Geometry: see drawing. Coordinates: mm, zero at the bounding-box minimum. A direction names the side the tool comes from. Coordinates: 2 decimals unless noted, no trailing zeros. Write each loop counter-clockwise with the first axis right and the second up, starting at its lowest first coordinate (ties: lowest second). Pieces come first, ordered by that corner, then holes.
1) Section query B-B (x = 16). Output: boundary loops of the cut face in (y, z) (1 decimal), then the cut area to 3 significant figures.
2) Section query A-A (z = 13). Output: boundary loops of the cut face in (x, y) (1 decimal).
3) Pin query (flat end, axial travel): pin 1 Ø10 at (y, z) = (96, 25) entering from +X; pin 2 Ø12 at (x, y) = (5, 98) entering from +Z (1 decimal); pin 3 Ø12 at (y, z) = (90.5, 12) entering from -X. Return the tip coordinate at first contact, or that it passes through.
4) Section query C-C (y = 111.5). Output: boundary loops of the cut face in (x, z), then the cut area to 3 significant figures.
5) Line query: L1, parallel to Y at x = 30, z = 30.5 (1 decimal); L2, parallel to X at y = 35.5, z = 25.5 (1 decimal); L3, parallel to X at y = 111, z = 22 (1 decimal). Output: solid intervals per line, ascending.
6) Set-up query: the marked faces 1 and 2. Return all of +Z, -Z, +X, -X, +Y, -Y with unobstructed straight access to the full face (end or side cutting, diameter ignored); none if empty.
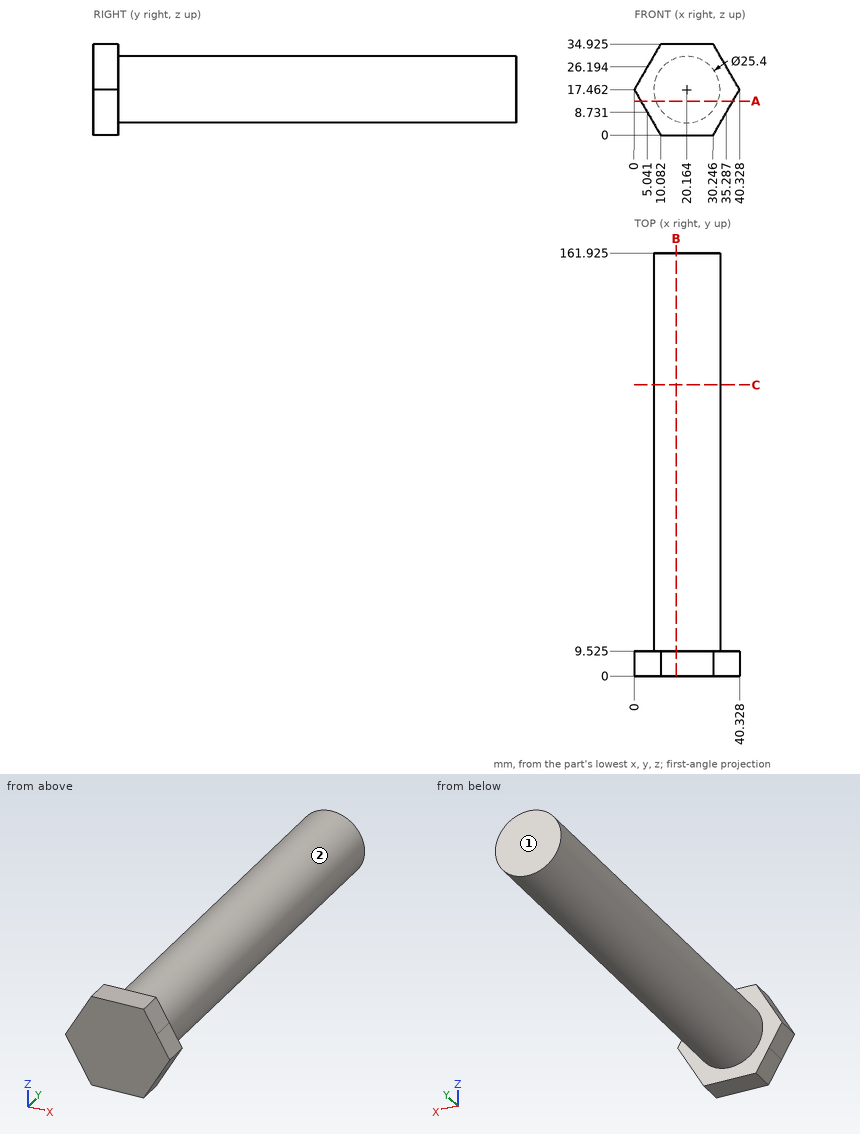
Answer:
1. outline: (0, 0) - (9.5, 0) - (9.5, 5.5) - (161.9, 5.5) - (161.9, 29.5) - (9.5, 29.5) - (9.5, 34.9) - (0, 34.9) - close
1. area: 3,990 mm2
2. outline: (2.6, 0) - (37.8, 0) - (37.8, 9.5) - (32.1, 9.5) - (32.1, 161.9) - (8.3, 161.9) - (8.3, 9.5) - (2.6, 9.5) - close
3. pin 1: stops at x = 32.61
3. pin 2: stops at z = 26.3
3. pin 3: stops at x = 7.46
4. outline: circle Ø25.4 at (20.16, 17.46)
4. area: 507 mm2
5. L1: y = 0 to 9.5
5. L2: x = 10.3 to 30
5. L3: x = 8.3 to 32
6. face 1: +Z, -Z, +X, -X, +Y
6. face 2: +Y
